Input: part model. Units: mm. Frame: model coordinates. Coordinates: 2 decimals unless noted, no trailing zeros. Loops run counter-clockwise (first coordinate to the right, second up) from the corner with the lowest first, then second, coordinate; pieces in that order, holes last. Notation, with made-up numbers: (30, 41.25) - (38, 41.25) arc R14 ccw to (38, 46.25) - close; hole circle Ø6 at (-17.75, 19). An arc over 180 degrees is marked (long way). Write item = value, one per line. Start each with the question number.
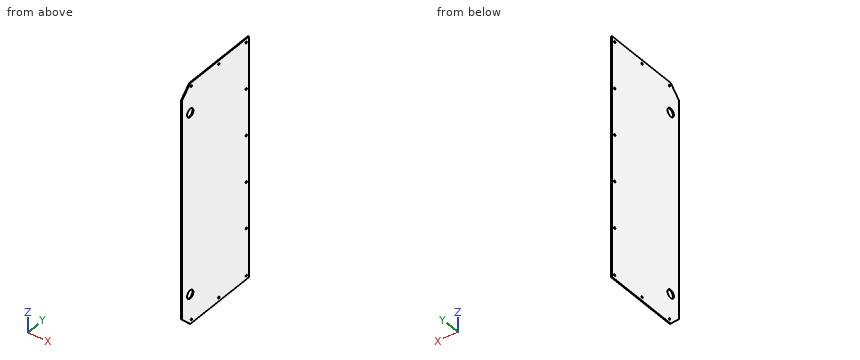
from build123d import *

# Parameters (mm, degrees)
SKETCH1_W          = 3.175
SKETCH1_H          = 304.8
BASE_FLANGE1_DEPTH = 412.75
SKETCH6_R          = 14.2875
SKETCH6_R_2        = 3.175
CUT_EXTRUDE1_DEPTH = 514.103969118


# Sheet-metal steps are written as plain solids
with BuildPart() as part:
    # Sketch1 → Base-Flange1 (new, symmetric)
    with BuildSketch(Plane.XY):
        with Locations((1.5875, 152.4)):
            Rectangle(SKETCH1_W, SKETCH1_H)
    extrude(amount=BASE_FLANGE1_DEPTH, both=True)

    # Sketch6 → Cut-Extrude1 (cut, through all)
    with BuildSketch(Plane(origin=(3.175, 0, 0), x_dir=(0, 0, -1), z_dir=(1, 0, 0))):
        with Locations((-311.15, 38.1)):
            Circle(SKETCH6_R)
        with Locations((311.15, 38.1)):
            Circle(SKETCH6_R)
        with Locations((-400.05, 292.1)):
            Circle(SKETCH6_R_2)
        with Locations((-400.05, 167.730256121)):
            Circle(SKETCH6_R_2)
        with Locations((-400.05, 43.360512242)):
            Circle(SKETCH6_R_2)
        with Locations(Location((400.05, 43.360512242, 0), (0, 0, 180))):
            Circle(SKETCH6_R_2)
        with Locations(Location((400.05, 292.1, 0), (0, 0, 180))):
            Circle(SKETCH6_R_2)
        with Locations(Location((400.05, 167.730256121, 0), (0, 0, 180))):
            Circle(SKETCH6_R_2)
        with Locations((-240.50625, 292.1)):
            Circle(SKETCH6_R_2)
        with Locations((-80.9625, 292.1)):
            Circle(SKETCH6_R_2)
        with Locations((78.58125, 292.1)):
            Circle(SKETCH6_R_2)
        with Locations((238.125, 292.1)):
            Circle(SKETCH6_R_2)
        Polygon((-412.75, 38.1), (-374.65, 0), (-412.75, 0), align=None)
        Polygon((412.75, 0), (412.75, 38.1), (374.65, 0), align=None)
    extrude(amount=-CUT_EXTRUDE1_DEPTH, mode=Mode.SUBTRACT)


solid = part.part
Item 1: Cut plane A-A on z = -311.15. Return loops of the section in (x, y) (1 decimal), plus the area to 3 significant figures.
Item 2: Pin query (flat end, axial travel): pin 1 (17 mm diameter, centred on y = 38.1, z = 311.15, fed in from +X); pin 2 (7.5 mm diameter, centred on y = 292.1, z = 80.96, fed in from +X) (3 decimals). Return the tip coordinate at first contact, or that it passes through.
Item 3: Ray query, line 1 (Y direction, x = 0.8, z = -400.05) (3 decimals); line 2 (Z direction, x = 2.75, y = 25.5); line 3 (Y direction, x = 1.1, z = -79.5). Return the intervals inside material, ascending.
Item 4: Cut plane B-B on z = 309.5. Return loops of the section in (x, y) (3 decimals).
Recorded:
q1.outline = (0, 0) - (3.2, 0) - (3.2, 23.8) - (0, 23.8) - close; (0, 52.4) - (3.2, 52.4) - (3.2, 304.8) - (0, 304.8) - close
q1.area = 877 mm²
q2.pin_1 = through
q2.pin_2 = 3.175
q3.line_1 = 25.4 to 40.186, 46.536 to 164.555, 170.905 to 288.925, 295.275 to 304.8
q3.line_2 = -400.15 to -317.89, -304.41 to 304.41, 317.89 to 400.15
q3.line_3 = 0 to 289.06, 295.14 to 304.8
q4.outline = (0, 0) - (3.175, 0) - (3.175, 23.908) - (0, 23.908) - close; (0, 52.292) - (3.175, 52.292) - (3.175, 304.8) - (0, 304.8) - close
